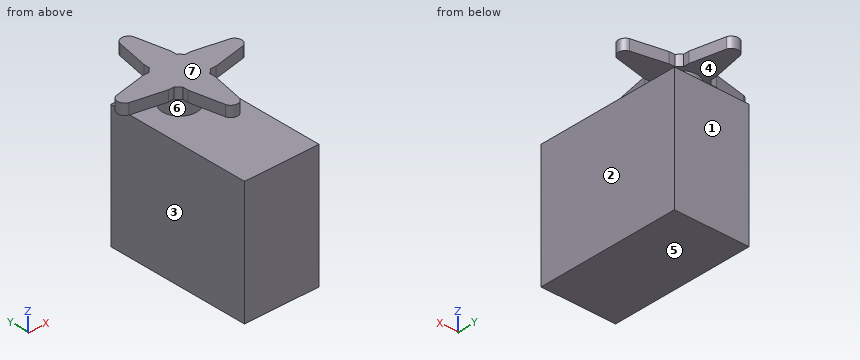
from build123d import *

# Parameters (mm, degrees)
F0_W     = 22
F0_H     = 42.5
F1_DEPTH = 36.6
F2_R     = 5
F3_DEPTH = 8.5
F6_DEPTH = 3.175
F7_DEPTH = 3.175
F8_COUNT = 4


with BuildPart() as f1:
    # F0 (on Top) → F1 (new body)
    with BuildSketch(Plane.XY):
        with Locations((11, 21.25)):
            Rectangle(F0_W, F0_H)
    extrude(amount=F1_DEPTH)

    # F2 (on face) → F3 (join)
    with BuildSketch(Plane.XY.offset(36.6)):
        with Locations((11, 32.5)):
            Circle(F2_R)
    extrude(amount=F3_DEPTH)

    # F5 (on offset) → F6 (join)
    with BuildSketch(Plane.XY.offset(45.1)):
        with BuildLine():
            ThreePointArc((7, 37.8124852941), (8.0316250237, 26.5492647513), (17.65, 32.5))
            ThreePointArc((17.65, 32.5), (16.9507352487, 35.4683749763), (15, 37.8124852941))
            Line((15, 37.8124852941), (7, 37.8124852941))
        make_face()
        with BuildLine():
            Line((7, 37.8124852941), (15, 37.8124852941))
            ThreePointArc((15, 37.8124852941), (11, 39.15), (7, 37.8124852941))
        make_face()
    extrude(amount=-F6_DEPTH)



with BuildPart() as f7:
    # F5 (on offset) → F7 (new body)
    with BuildSketch(Plane.XY.offset(45.1)):
        with BuildLine():
            ThreePointArc((7, 37.8124852941), (11, 39.15), (15, 37.8124852941))
            Line((15, 37.8124852941), (15, 39.5))
            Line((15, 39.5), (13, 49.3124852941))
            ThreePointArc((13, 49.3124852941), (11, 50.8124852941), (9, 49.3124852941))
            Line((9, 49.3124852941), (7, 39.5))
            Line((7, 39.5), (7, 37.8124852941))
        make_face()
    extrude(amount=-F7_DEPTH)


with BuildPart() as f1_1:
    add(f1.part)

    add(f7.part)  # F8 merges F7
    # F8: F7 ×4 about axis
    f8_axis = Axis((11, 32.5, 45.1), (0, 0, 1))
    for i in range(1, F8_COUNT):
        add(f7.part.rotate(f8_axis, i * 360 / F8_COUNT))


solid = f1_1.part
Model file for the job. Use its own axes, mm. Face numbers are marked on the shaded views. A direction names the side the tool comes from. Give positions to 0.01 mm unless a question says otherwise; leave off trailing zeros. Loops run counter-clockwise (first coordinate to the right, second up) from the corner with the lowest first, then second, coordinate; pieces in that order, holes last.
Item 1: Mould opens along Z. For the marked faces 5, 6 and 7 say: +Z half, -Z half, draft (parallel to the pull), parting line (faces both ways), or undercut.
Check values:
face 5: -Z half
face 6: undercut
face 7: +Z half
Item 2: Slice it at A-A (y = 38.5). Write the cut outline in (x, z) (3 decimals), plus the area to 3 significant figures.
Check values:
outline: (0, 0) - (22, 0) - (22, 36.6) - (0, 36.6) - close; (7, 41.925) - (15, 41.925) - (15, 45.1) - (7, 45.1) - close
area: 831 mm2
Item 3: Slice it at C-C (y = 32.5). Write the cut outline in (x, z) (3 decimals), plus the area to 3 significant figures.
Check values:
outline: (-7.312, 41.925) - (6, 41.925) - (6, 36.6) - (0, 36.6) - (0, 0) - (22, 0) - (22, 36.6) - (16, 36.6) - (16, 41.925) - (29.312, 41.925) - (29.312, 45.1) - (-7.312, 45.1) - close
area: 975 mm2
Item 4: Slice it at B-B (x = 11). Write the cut outline in (y, z) (3 decimals).
Check values:
outline: (0, 0) - (42.5, 0) - (42.5, 36.6) - (37.5, 36.6) - (37.5, 41.925) - (50.812, 41.925) - (50.812, 45.1) - (14.188, 45.1) - (14.188, 41.925) - (27.5, 41.925) - (27.5, 36.6) - (0, 36.6) - close
Item 5: Slice it at D-D (z = 37.5). Write the cut outline in (x, y).
Check values:
outline: circle Ø10 at (11, 32.5)
Item 6: Which spindle directions (+Z, -Z, +X, -X, +Y, -Y) get a long thin tool onto all of the face, cutting with end or side? Do the marked faces 1, 2, 3 and 4. Say none if no direction does.
Check values:
face 1: -Z, +X, -X, +Y
face 2: -Z, +X, +Y, -Y
face 3: -Z, -X, +Y, -Y
face 4: none
Item 7: Drop flat-ended pins along their axis: P1, Ø5, axis at y = 31.5, z = 25, coming from the +X side; P2, Ø6, axis at x = 14.5, z = 21, coming from the +Y side; P3, Ø1.9, axis at x = 5, z = 43.5, coming from the +Y side; P4, Ø1, axis at x = -2.5, z = 39.5, coming from the +Y side. Give the stop position or say it passes through.
Check values:
P1: stops at x = 22
P2: stops at y = 42.5
P3: stops at y = 36.83
P4: passes through
Item 8: Drill centre lines: line 1 along Z through (x, y) = (20.5, 33.5) (3 decimals); line 2 along Y through (x, z) = (5, 7.5); line 3 along X through (y, z) = (27, 13). Where is each one in solid material? Low to high.
Check values:
line 1: z = 0 to 36.6, 41.925 to 45.1
line 2: y = 0 to 42.5
line 3: x = 0 to 22
